from build123d import *

# Parameters (mm, degrees)
SKETCH1_W           = 370
SKETCH1_H           = 200
BOSS_EXTRUDE1_DEPTH = 15
SKETCH2_W           = 28.561692334
SKETCH2_H           = 200
SKETCH2_W_2         = 30
BOSS_EXTRUDE2_DEPTH = 200
SKETCH3_R           = 20
CUT_EXTRUDE1_DEPTH  = 200


with BuildPart() as part:
    # Sketch1 → Boss-Extrude1 (new body)
    with BuildSketch(Plane(origin=(0, 0, 0), x_dir=(1, 0, 0), z_dir=(0, 1, 0))):
        Rectangle(SKETCH1_W, SKETCH1_H)
    extrude(amount=BOSS_EXTRUDE1_DEPTH)

    # Sketch2 → Boss-Extrude2 (add)
    with BuildSketch(Plane.XZ):
        with Locations((-170.719153833, 0)):
            Rectangle(SKETCH2_W, SKETCH2_H)
        with Locations((170, 0)):
            Rectangle(SKETCH2_W_2, SKETCH2_H)
    extrude(amount=BOSS_EXTRUDE2_DEPTH)

    # Sketch3 → Cut-Extrude1 (cut)
    with BuildSketch(Plane(origin=(0, 15, 0), x_dir=(1, 0, 0), z_dir=(0, 1, 0))):
        with Locations(Location((0, 0, 0), (0, 0, 270))):
            Circle(SKETCH3_R)
    extrude(amount=-CUT_EXTRUDE1_DEPTH, mode=Mode.SUBTRACT)


solid = part.part
Can you work these out from the model? Positions are in its coordinate system, mm. A direction names the side the tool comes from. Coordinates: 2 decimals unless noted, no trailing zeros. Loops run counter-clockwise (first coordinate to the right, second up) from the corner with the lowest first, then second, coordinate; pieces in that order, holes last. Notation, with made-up numbers: (-17.75, -33) - (34.25, -33) arc R36 ccw to (34.25, 1) - close; hole circle Ø7 at (9, -23.75). An arc over 180 degrees is marked (long way). Put each result on its own line as item: value. Start each with the question number.
Item 1: If we mould it in two halves opening along X, with no side actions, what happens to faces 1 (the face through (-185, -91, -1)), 2 (the face through (-156.438, -99, -1)), 3 (the face through (170, -200, 1))? For each: +X half, -X half, draft (parallel to the pull), parting line (faces both ways), or undercut.
Item 2: Suppose I cut it at D-D (z = 81). Please give me the cut outline in (x, y).
Item 3: Suppose I cut it at B-B (z = 0). Please give me the cut outline in (x, y).
Item 4: If I drill on line 1 along X through (y, z) = (5, 0); line 2 along X through (y, z) = (-184.5, 16); line 3 along Y through (x, z) = (-76, -49), over which ranges is the centre line in solid material (lowest first)?
Item 5: Which directions (+Z, -Z, +X, -X, +Y, -Y) give clear straight access to the entire face, cutting with the end or side of a thin tool? Please do faces 4 (the face through (-171, -200, 1)), 5 (the face through (155, -99, -1)).
Item 6: Suppose I cut it at A-A (y = -60). Please give me the cut outline in (x, z).
Item 7: Suppose I cut it at C-C (x = 0). Please give me the cut outline in (y, z), and give its area (3 significant figures).
Here are the results:
1. face 1: -X half
1. face 2: undercut
1. face 3: draft
2. outline: (-185, -200) - (-156.44, -200) - (-156.44, 0) - (155, 0) - (155, -200) - (185, -200) - (185, 15) - (-185, 15) - close
3. outline: (-185, -200) - (-156.44, -200) - (-156.44, 0) - (-20, 0) - (-20, 15) - (-185, 15) - close; (20, 0) - (155, 0) - (155, -200) - (185, -200) - (185, 15) - (20, 15) - close
4. line 1: -185 to -20, 20 to 185
4. line 2: -185 to -156.44, 155 to 185
4. line 3: 0 to 15
5. face 4: +Z, -Z, +X, -X, -Y
5. face 5: +Z, -Z, -Y
6. outline: (-185, -100) - (-156.44, -100) - (-156.44, 100) - (-185, 100) - close; (155, -100) - (185, -100) - (185, 100) - (155, 100) - close
7. outline: (0, -100) - (15, -100) - (15, -20) - (0, -20) - close; (0, 20) - (15, 20) - (15, 100) - (0, 100) - close
7. area: 2,400 mm²
